```python
from build123d import *

# Parameters (mm, degrees)
SKETCH2_OUTSIDE_W  = 25.754
SKETCH2_OUTSIDE_H  = 25.754
SKETCH2_OUTSIDE_R  = 2.5527
CUT_EXTRUDE3_DEPTH = 48.090483291
CHAMFER1_SIZE      = 0.254


with BuildPart() as part:
    # Sketch1 → Revolve1 (revolve)
    with BuildSketch(Plane(origin=(0, 0, 0), x_dir=(0, 0, -1), z_dir=(1, 0, 0))):
        Polygon((0, 0), (-46.0756, 0), (-46.0756, 6.35), (-34.6075, 6.35), (-34.6075, 6.87578), (-9.3091, 6.87578), (-9.3091, 6.35), (0, 6.35), align=None)
    revolve(axis=Axis((0, 0, -29.540514156), (0, 0, 1)))

    # Sketch2 outside → Cut-Extrude3 (cut, through all)
    # profile 1 of 2: a face of its own
    with BuildSketch(Plane(origin=(0, 0, 0), x_dir=(-1, 0, 0), z_dir=(0, 0, -1))):
        Rectangle(SKETCH2_OUTSIDE_W, SKETCH2_OUTSIDE_H)
        Polygon((3.666174209, -6.35), (7.332348419, 0), (3.666174209, 6.35), (-3.666174209, 6.35), (-7.332348419, 0), (-3.666174209, -6.35), align=None, mode=Mode.SUBTRACT)
    # profile 2 of 2: a face of its own
    with BuildSketch(Plane(origin=(0, 0, 0), x_dir=(-1, 0, 0), z_dir=(0, 0, -1))):
        Circle(SKETCH2_OUTSIDE_R)
    extrude(amount=-CUT_EXTRUDE3_DEPTH, mode=Mode.SUBTRACT)

    # Chamfer1
    chamfer1_edges = [part.edges().sort_by_distance(p)[0] for p in [
        (0, -6.35, 0),
        (0, -6.35, 46.0756),
    ]]
    chamfer(chamfer1_edges, length=CHAMFER1_SIZE)


solid = part.part
```
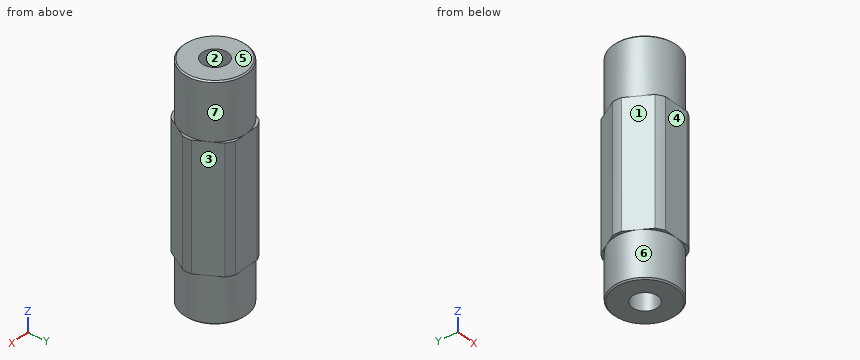
Can you work these out from the model? Positions are in its coordinate system, mm. Face numbers are marked on the shaded views. A direction names the side the tool comes from. Give positions to 0.01 mm unless a question says otherwise; leave off trailing zeros. Order: outer loops, then holes, each group sorted by start corner. A loop starts at its lowest first (then second) coordinate and runs counter-clockwise, first axis right, second up. Notation, with made-up numbers: M -35,46 L -11,46 A11 cw -11,60 Z; hole C 3.5,63.5 d9. An arc over 180 degrees is marked long. One line per item, written item: value.
1) For P1, Ø1.5, axis at y = 4, z = 21, coming from the -X side; P2, Ø6, axis at y = 5, z = 9.5, coming from the +X side; P3, Ø3, axis at y = 4.5, z = 16, coming from the +X side, each with a flat end and sliding along its axis, tell me the tip position at first contact or that it passes through.
Answer sheet:
P1: stops at x = -5.46
P2: stops at x = 6.18
P3: stops at x = 5.6
2) On a 3-axis mill with a long thin cutter (end or side, diameter ignored), from which of +Z, -Z, +X, -X, +Y, -Y can I reach the whole of each face in a straight line? I mean the marked faces 5, 6 and 7. Say none if no direction works.
Answer sheet:
face 5: +Z, +X, -X, +Y, -Y
face 6: -Z
face 7: +Z
3) I want a section at C-C, the plane z = 5.5. List the corners of the cut face in (x, y) for me.
Answer sheet:
outline: C 0,0 d12.7; hole C 0,0 d5.11
4) I want a section at A-A, the plane y = 0. List the corners of the cut face in (x, z) for me, plus the area to 3 significant figures.
Answer sheet:
outline: M -6.88,9.31 L -6.35,9.31 L -6.35,0.25 L -6.1,0 L -2.55,0 L -2.55,46.08 L -6.1,46.08 L -6.35,45.82 L -6.35,34.61 L -6.88,34.61 Z; M 2.55,0 L 6.1,0 L 6.35,0.25 L 6.35,9.31 L 6.88,9.31 L 6.88,34.61 L 6.35,34.61 L 6.35,45.82 L 6.1,46.08 L 2.55,46.08 Z
area: 376 mm^2
5) Please list where these lines run through material, in increasing order: line 1 along Y through (x, z) = (0, 24); line 2 along Z through (x, y) = (4, -5).
Answer sheet:
line 1: y = -6.35 to -2.55, 2.55 to 6.35
line 2: z = 9.31 to 34.61
6) We'd pull the mould along X, two halves only. Please class the marked faces 1, 2, 3 and 4: released by +X, released by -X, zero draft, split by the parting line, or undercut.
Answer sheet:
face 1: released by -X
face 2: undercut
face 3: released by +X
face 4: zero draft
7) I want a section at B-B, the plane z = 34. List the corners of the cut face in (x, y) for me.
Answer sheet:
outline: M -6.82,-0.89 L -4.18,-5.46 A6.88 ccw -2.64,-6.35 L 2.64,-6.35 A6.88 ccw 4.18,-5.46 L 6.82,-0.89 A6.88 ccw 6.82,0.89 L 4.18,5.46 A6.88 ccw 2.64,6.35 L -2.64,6.35 A6.88 ccw -4.18,5.46 L -6.82,0.89 A6.88 ccw Z; hole C 0,0 d5.11
